```python
from build123d import *

# Parameters (mm, degrees)
CHAMFER_1_SIZE = 0.5


with BuildPart() as part:
    # 草图1 → 旋转1 (revolve)
    with BuildSketch(Plane.XY, mode=Mode.PRIVATE) as revolve_1_sk:
        Polygon((14, 0), (14, 2), (15, 2), (15, 7), (16.15, 7), (16.15, 8), (15, 8), (15, 16), (17.65, 16), (17.65, 17), (16.5, 17), (16.5, 21.5), (18.55, 21.5), (19.05, 21), (19.05, 5.5), (18.55, 5), (17, 5), (17, 4), (18.5, 4), (18.5, 0.5), (18, 0), align=None)
    revolve(revolve_1_sk.sketch.rotate(Axis((0, 0, 0), (0, 1, 0)), 90), axis=Axis((0, 0, 0), (0, 1, 0)))  # turned: the seam where the file's is

    # 倒角1
    chamfer_1_edges = [part.edges().sort_by_distance(p)[0] for p in [
        (0, 16, 15),
        (0, 21.5, 16.5),
    ]]
    chamfer(chamfer_1_edges, length=CHAMFER_1_SIZE)


solid = part.part
```
Geometry check sheet. Reference: the model listing, model coordinates, mm. A direction names the side the tool comes from. Give positions to 0.01 mm unless a question says otherwise; leave off trailing zeros. Write each loop counter-clockwise with the first axis right and the second up, starting at its lowest first coordinate (ties: lowest second). Pieces come first, ordered by that corner, then holes.
1) Gauge pin test, flat ends, axial feed: pin 1 (4 mm diameter, centred on y = 15, z = 15, fed in from -X); pin 2 (1 mm diameter, centred on x = -13, y = 2.5, fed in from -Z); pin 3 (15 mm diameter, centred on x = -6.5, z = -3.5, fed in from +Y). Record the tip position at first contact, or that the pin passes through.
2) Release check for a two-part mould opening along Z. For faces 5 (the cylindrical face through (18.597, 13.142, 4.13)), 6 (the flat face through (5.4, 5, -16.4)), 7 (the cylindrical face through (17.23, 16.51, 3.83)), 8 (the cylindrical face through (-12.65, 4.54, -8.06)) record: pulls with the +Z half, pulls with the -Z half, needs draft (parallel to the pull), parting line crosses it, or undercut.
3) Access from +Z, -Z, +X, -X, +Y, -Y to the whole of each face (thin tool, end or side, straight path). Record for faces 1 (the flat face through (12, 17, -12)), 2 (the cylindrical face through (16.41, 2.23, -8.54)), 3 (the flat face through (5.4, 21.5, 16.4)), 4 (the cylindrical face through (-4.956, 19.028, -15.738)).
4) Section check A-A, the plane y = 18.75. Record the boundary of the cut face in (x, z), and give its area (3 significant figures).
5) Material ranges on L1, parallel to X at y = 16.7, z = 0; L2, parallel to Y at x = -15.5, z = 4; L3, parallel to X at y = 3.55, z = 0, recorded low to high.
Computed:
1. pin 1: stops at x = -13.92
1. pin 2: stops at z = -13.64
1. pin 3: stops at y = 2
2. face 5: parting line crosses it
2. face 6: needs draft
2. face 7: undercut
2. face 8: undercut
3. face 1: none
3. face 2: -Y
3. face 3: +Z, -Z, +X, -X, +Y
3. face 4: +Y
4. outline: circle Ø38.1 at (0, 0); hole circle Ø33 at (0, 0)
4. area: 285 mm2
5. L1: x = -19.05 to -17.65, 17.65 to 19.05
5. L2: y = 0 to 7, 8 to 16
5. L3: x = -18.5 to -15, 15 to 18.5
